```python
from build123d import *

# Parameters (mm, degrees)
ESQUISSE1_W              = 60
ESQUISSE1_H              = 89
BOSS_EXTRU_1_DEPTH       = 11.5
ESQUISSE2_W              = 15
ESQUISSE2_H              = 1.6
ENL_V_MAT_EXTRU_1_DEPTH  = 55.886246
ENL_V_MAT_EXTRU_2_REACH  = 94.584
ESQUISSE4_W              = 15
ESQUISSE4_H              = 9.9
ENL_V_MAT_EXTRU_3_REACH  = 75.647
ESQUISSE5_W              = 85.8
ESQUISSE5_H              = 9.9
ENL_V_MAT_EXTRU_4_REACH  = 75.647
ESQUISSE6_W              = 9.9
ESQUISSE6_H              = 85.8
ENL_V_MAT_EXTRU_5_REACH  = 76.922
ESQUISSE7_W              = 7
ESQUISSE7_H              = 10
ENL_V_MAT_EXTRU_6_REACH  = 76.922
ESQUISSE8_W              = 7
ESQUISSE8_H              = 18
ENL_V_MAT_EXTRU_7_REACH  = 96.096
ESQUISSE9_W              = 17.5
ESQUISSE9_H              = 7.5
ENL_V_MAT_EXTRU_8_REACH  = 96.096
ESQUISSE10_W             = 16
ESQUISSE10_H             = 7.5
ENL_V_MAT_EXTRU_9_REACH  = 96.096
ESQUISSE11_W             = 16
ESQUISSE11_H             = 7.5
ENL_V_MAT_EXTRU_10_REACH = 76.922
ESQUISSE12_W             = 7
ESQUISSE12_H             = 8.5
ESQUISSE23_W             = 2
ESQUISSE23_H             = 7.5
BOSS_EXTRU_5_DEPTH       = 7.5
ESQUISSE24_W             = 7.5
ESQUISSE24_H             = 2
BOSS_EXTRU_6_DEPTH       = 7.5
ESQUISSE25_W             = 2
ESQUISSE25_H             = 7.5
BOSS_EXTRU_7_DEPTH       = 8.1
ESQUISSE26_W             = 2
ESQUISSE26_H             = 7.5
BOSS_EXTRU_8_DEPTH       = 7.5
ESQUISSE28_W             = 1.25
ESQUISSE28_H             = 7
ESQUISSE29_W             = 1.25
ESQUISSE29_H             = 7
ESQUISSE30_W             = 1.25
ESQUISSE30_H             = 7
ESQUISSE31_W             = 1.25
ESQUISSE31_H             = 7
CONG_1_R                 = 2
CHANFREIN1_SIZE          = 0.3
CONG_2_R                 = 0.5
CONG_9_R                 = 2.5


with BuildPart() as part:
    # Esquisse1 → Boss.-Extru.1 (new body)
    with BuildSketch(Plane.XY.offset(5.75)):
        Rectangle(ESQUISSE1_W, ESQUISSE1_H)
    extrude(amount=-BOSS_EXTRU_1_DEPTH)

    # Esquisse2 → Enlèv. mat.-Extru.1 (cut, through all)
    with BuildSketch(Plane(origin=(0, 0, -5.75), x_dir=(-1, 0, 0), z_dir=(0, 0, -1))):
        with Locations((0, 43.7)):
            Rectangle(ESQUISSE2_W, ESQUISSE2_H)
    extrude(amount=-ENL_V_MAT_EXTRU_1_DEPTH, mode=Mode.SUBTRACT)

    # Esquisse4 → Enlèv. mat.-Extru.2 (cut, up to next)
    with BuildSketch(Plane.XZ.offset(42.9), mode=Mode.PRIVATE) as enl_v_mat_extru_2_sk1:
        with Locations((0, 0.8)):
            Rectangle(ESQUISSE4_W, ESQUISSE4_H)
    enl_v_mat_extru_2_tool1 = extrude(enl_v_mat_extru_2_sk1.sketch, amount=-ENL_V_MAT_EXTRU_2_REACH, mode=Mode.PRIVATE) & part.part
    add(enl_v_mat_extru_2_tool1.solids().sort_by_distance((0, -42.9, 0.8))[0], mode=Mode.SUBTRACT)

    # Esquisse5 → Enlèv. mat.-Extru.3 (cut, up to next)
    with BuildSketch(Plane(origin=(-28.4, 0, 0), x_dir=(0, -1, 0), z_dir=(-1, 0, 0)), mode=Mode.PRIVATE) as enl_v_mat_extru_3_sk1:
        with Locations((0, 0.8)):
            Rectangle(ESQUISSE5_W, ESQUISSE5_H)
    enl_v_mat_extru_3_tool1 = extrude(enl_v_mat_extru_3_sk1.sketch, amount=-ENL_V_MAT_EXTRU_3_REACH, mode=Mode.PRIVATE) & part.part
    add(enl_v_mat_extru_3_tool1.solids().sort_by_distance((-28.4, 0, 0.8))[0], mode=Mode.SUBTRACT)

    # Esquisse6 → Enlèv. mat.-Extru.4 (cut, up to next)
    with BuildSketch(Plane(origin=(28.4, 0, 0), x_dir=(0, 0, -1), z_dir=(1, 0, 0)), mode=Mode.PRIVATE) as enl_v_mat_extru_4_sk1:
        with Locations((-0.8, 0)):
            Rectangle(ESQUISSE6_W, ESQUISSE6_H)
    enl_v_mat_extru_4_tool1 = extrude(enl_v_mat_extru_4_sk1.sketch, amount=-ENL_V_MAT_EXTRU_4_REACH, mode=Mode.PRIVATE) & part.part
    add(enl_v_mat_extru_4_tool1.solids().sort_by_distance((28.4, 0, 0.8))[0], mode=Mode.SUBTRACT)

    # Esquisse7 → Enlèv. mat.-Extru.5 (cut, up to next)
    with BuildSketch(Plane.ZY.offset(30), mode=Mode.PRIVATE) as enl_v_mat_extru_5_sk1:
        with Locations((2.25, 32)):
            Rectangle(ESQUISSE7_W, ESQUISSE7_H)
    enl_v_mat_extru_5_tool1 = extrude(enl_v_mat_extru_5_sk1.sketch, amount=-ENL_V_MAT_EXTRU_5_REACH, mode=Mode.PRIVATE) & part.part
    add(enl_v_mat_extru_5_tool1.solids().sort_by_distance((-30, 32, 2.25))[0], mode=Mode.SUBTRACT)

    # Esquisse8 → Enlèv. mat.-Extru.6 (cut, up to next)
    with BuildSketch(Plane.ZY.offset(30), mode=Mode.PRIVATE) as enl_v_mat_extru_6_sk1:
        with Locations((2.25, 10.5)):
            Rectangle(ESQUISSE8_W, ESQUISSE8_H)
    enl_v_mat_extru_6_tool1 = extrude(enl_v_mat_extru_6_sk1.sketch, amount=-ENL_V_MAT_EXTRU_6_REACH, mode=Mode.PRIVATE) & part.part
    add(enl_v_mat_extru_6_tool1.solids().sort_by_distance((-30, 10.5, 2.25))[0], mode=Mode.SUBTRACT)

    # Esquisse9 → Enlèv. mat.-Extru.7 (cut, up to next)
    with BuildSketch(Plane.XZ.offset(44.5), mode=Mode.PRIVATE) as enl_v_mat_extru_7_sk1:
        with Locations((-17.75, 2)):
            Rectangle(ESQUISSE9_W, ESQUISSE9_H)
    enl_v_mat_extru_7_tool1 = extrude(enl_v_mat_extru_7_sk1.sketch, amount=-ENL_V_MAT_EXTRU_7_REACH, mode=Mode.PRIVATE) & part.part
    add(enl_v_mat_extru_7_tool1.solids().sort_by_distance((-17.75, -44.5, 2))[0], mode=Mode.SUBTRACT)

    # Esquisse10 → Enlèv. mat.-Extru.8 (cut, up to next)
    with BuildSketch(Plane.XZ.offset(44.5), mode=Mode.PRIVATE) as enl_v_mat_extru_8_sk1:
        with Locations((1, 2)):
            Rectangle(ESQUISSE10_W, ESQUISSE10_H)
    enl_v_mat_extru_8_tool1 = extrude(enl_v_mat_extru_8_sk1.sketch, amount=-ENL_V_MAT_EXTRU_8_REACH, mode=Mode.PRIVATE) & part.part
    add(enl_v_mat_extru_8_tool1.solids().sort_by_distance((1, -44.5, 2))[0], mode=Mode.SUBTRACT)

    # Esquisse11 → Enlèv. mat.-Extru.9 (cut, up to next)
    with BuildSketch(Plane.XZ.offset(44.5), mode=Mode.PRIVATE) as enl_v_mat_extru_9_sk1:
        with Locations((19, 2)):
            Rectangle(ESQUISSE11_W, ESQUISSE11_H)
    enl_v_mat_extru_9_tool1 = extrude(enl_v_mat_extru_9_sk1.sketch, amount=-ENL_V_MAT_EXTRU_9_REACH, mode=Mode.PRIVATE) & part.part
    add(enl_v_mat_extru_9_tool1.solids().sort_by_distance((19, -44.5, 2))[0], mode=Mode.SUBTRACT)

    # Esquisse12 → Enlèv. mat.-Extru.10 (cut, up to next)
    with BuildSketch(Plane.ZY.offset(30), mode=Mode.PRIVATE) as enl_v_mat_extru_10_sk1:
        with Locations((2.25, -11)):
            Rectangle(ESQUISSE12_W, ESQUISSE12_H)
    enl_v_mat_extru_10_tool1 = extrude(enl_v_mat_extru_10_sk1.sketch, amount=-ENL_V_MAT_EXTRU_10_REACH, mode=Mode.PRIVATE) & part.part
    add(enl_v_mat_extru_10_tool1.solids().sort_by_distance((-30, -11, 2.25))[0], mode=Mode.SUBTRACT)

    # Esquisse23 → Boss.-Extru.5 (add)
    with BuildSketch(Plane(origin=(-28.4, 0, 0), x_dir=(0, 0, -1), z_dir=(1, 0, 0))):
        with Locations((3.15, 39.15)):
            Rectangle(ESQUISSE23_W, ESQUISSE23_H)
    extrude(amount=BOSS_EXTRU_5_DEPTH)

    # Esquisse24 → Boss.-Extru.6 (add)
    with BuildSketch(Plane.XZ.offset(-42.9)):
        with Locations((24.65, -3.15)):
            Rectangle(ESQUISSE24_W, ESQUISSE24_H)
    extrude(amount=BOSS_EXTRU_6_DEPTH)

    # Esquisse25 → Boss.-Extru.7 (add)
    with BuildSketch(Plane.ZY.offset(-28.4)):
        with Locations((-3.15, -18.85)):
            Rectangle(ESQUISSE25_W, ESQUISSE25_H)
    extrude(amount=BOSS_EXTRU_7_DEPTH)

    # Esquisse26 → Boss.-Extru.8 (add)
    with BuildSketch(Plane(origin=(-28.4, 0, 0), x_dir=(0, 0, -1), z_dir=(1, 0, 0))):
        with Locations((3.15, -18.85)):
            Rectangle(ESQUISSE26_W, ESQUISSE26_H)
    extrude(amount=BOSS_EXTRU_8_DEPTH)

    # Esquisse28 → Révolution1 (revolve)
    with BuildSketch(Plane(origin=(0, -18.85, 0), x_dir=(1, 0, 0), z_dir=(0, 1, 0))):
        with Locations((24.975, -1.35)):
            Rectangle(ESQUISSE28_W, ESQUISSE28_H)
    revolve(axis=Axis((24.35, -18.85, -2.15), (0, 0, 1)))

    # Esquisse29 → Révolution2 (revolve)
    with BuildSketch(Plane(origin=(0, 39.15, 0), x_dir=(1, 0, 0), z_dir=(0, 1, 0))):
        with Locations((24.975, -1.35)):
            Rectangle(ESQUISSE29_W, ESQUISSE29_H)
    revolve(axis=Axis((24.35, 39.15, -2.15), (0, 0, 1)))

    # Esquisse30 → Révolution3 (revolve)
    with BuildSketch(Plane(origin=(0, 39.15, 0), x_dir=(1, 0, 0), z_dir=(0, 1, 0))):
        with Locations((-24.025, -1.35)):
            Rectangle(ESQUISSE30_W, ESQUISSE30_H)
    revolve(axis=Axis((-24.65, 39.15, -2.15), (0, 0, 1)))

    # Esquisse31 → Révolution4 (revolve)
    with BuildSketch(Plane(origin=(0, -18.85, 0), x_dir=(1, 0, 0), z_dir=(0, 1, 0))):
        with Locations((-24.025, -1.35)):
            Rectangle(ESQUISSE31_W, ESQUISSE31_H)
    revolve(axis=Axis((-24.65, -18.85, -2.15), (0, 0, 1)))

    # Congé1
    cong_1_edges = [part.edges().sort_by_distance(p)[0] for p in [
        (30, -44.5, 0),
        (-30, -44.5, 0),
        (-30, 44.5, 0),
        (30, 44.5, 0),
    ]]
    fillet(cong_1_edges, radius=CONG_1_R)

    # Chanfrein1
    chanfrein1_edges = [part.edges().sort_by_distance(p)[0] for p in [
        (23.1, -18.85, 4.85),
        (23.1, 39.15, 4.85),
        (-25.9, 39.15, 4.85),
        (-25.9, -18.85, 4.85),
    ]]
    chamfer(chanfrein1_edges, length=CHANFREIN1_SIZE)

    # Congé2
    cong_2_edges = [part.edges().sort_by_distance(p)[0] for p in [
        (-17.75, 44.5, -5.75),
        (30, 0, -5.75),
        (17.75, 44.5, -5.75),
        (0, -44.5, -5.75),
        (-30, 0, -5.75),
        (-29.414213562, -43.914213562, -5.75),
        (29.414213562, -43.914213562, -5.75),
        (-29.414213562, 43.914213562, -5.75),
        (29.414213562, 43.914213562, -5.75),
    ]]
    fillet(cong_2_edges, radius=CONG_2_R)

    # Congé9
    cong_9_edges = [part.edges().sort_by_distance(p)[0] for p in [
        (-28.4, 35.4, -3.15),
        (-20.9, 35.4, -3.15),
        (-20.9, 42.9, -3.15),
        (20.9, 42.9, -3.15),
        (20.9, 35.4, -3.15),
        (28.4, 35.4, -3.15),
        (28.4, -22.6, -3.15),
        (28.4, -15.1, -3.15),
        (20.3, -22.6, -3.15),
        (20.3, -15.1, -3.15),
        (-28.4, -22.6, -3.15),
        (-28.4, -15.1, -3.15),
        (-20.9, -22.6, -3.15),
        (-20.9, -15.1, -3.15),
    ]]
    fillet(cong_9_edges, radius=CONG_9_R)


solid = part.part
```
For this review, take the finished solid that the model builds, in its own axes (mm). A direction names the side the tool comes from. Coordinates: 2 decimals unless noted, no trailing zeros. Write each loop counter-clockwise with the first axis right and the second up, starting at its lowest first coordinate (ties: lowest second). Pieces come first, ordered by that corner, then holes. Notation, with made-up numbers: (-32, 28.25) - (-11, 28.25) arc R17 ccw to (-11, 46.25) - close; hole circle Ø4 at (71.5, 20.25). An arc over 180 degrees is marked (long way). Answer in a Markdown table with one row per item. Add a question column.
Q1. We need section C-C, the plane z = 1.75. Count the separate pieces of the cut face and the enclosed holes in it, and give its area (3 significant figures).
Q2. We need section B-B, the plane x = 13.5. State the section outline as (y, z) points, and give its area (3 significant figures).
Q3. Draft analysis for pull direction X (two halves, no side actions). For faces 3 (the flat face through (30, -1, 0)), 4 (the flat face through (-25, 39, 4.85)), 5 (the flat face through (18, 44.5, 0)), state which applies: +X half, -X half, draft (parallel to the pull), parting line (faces both ways), or undercut.
Q4. We need section D-D, the plane x = 24.35. State the section outline as (y, z) points, and give its area (3 significant figures).
Q5. For probe 1 along X at (y, z) = (16, -2.5); probe 2 along Y at (x, z) = (17, -4); probe 3 along Y at (x, z) = (-2.5, -4), list the stretches that pass through material, from the lowest coordinate up.
Q6. Tool access review of faces 1 (the cylindrical face through (-29.43, 43.9, 0.17)), 2 (the flat face through (20.9, 39, -3)): name each direction out of +Z, -Z, +X, -X, +Y, -Y from which nothing blocks a thin tool from reaching the whole face with its end or side.
Q7. For P1, Ø1.5, axis at x = -24, y = 39.5, coming from the +Z side; P2, Ø0.5, axis at x = -29.5, z = 2.5, coming from the +Y side; P3, Ø0.8, axis at x = -29.5, z = 0.5, coming from the -Y side, all flat-tipped, find the tip position at first contact; note any pin that passes through.
Q8. We need section A-A, the plane y = -27.5. State the section outline as (x, z) points, and give its area (3 significant figures).
Answer list:
| question | item | result |
|---|---|---|
| 1 | separate pieces | 11 |
| 1 | enclosed holes | 0 |
| 1 | area | 321 mm2 |
| 2 | outline | (-44.5, -5.25) arc R0.5 ccw to (-44, -5.75) - (44, -5.75) arc R0.5 ccw to (44.5, -5.25) - (44.5, 5.75) - (42.9, 5.75) - (42.9, -4.15) - (-42.9, -4.15) - (-42.9, -1.75) - (-44.5, -1.75) - close |
| 2 | area | 162 mm2 |
| 3 | face 3 | +X half |
| 3 | face 4 | undercut |
| 3 | face 5 | draft |
| 4 | outline | (-44.5, -5.25) arc R0.5 ccw to (-44, -5.75) - (44, -5.75) arc R0.5 ccw to (44.5, -5.25) - (44.5, 5.75) - (42.9, 5.75) - (42.9, -2.15) - (40.4, -2.15) - (40.4, 4.55) - (40.1, 4.85) - (38.2, 4.85) - (37.9, 4.55) - (37.9, -2.15) - (35.4, -2.15) - (35.4, -4.15) - (-15.1, -4.15) - (-15.1, -2.15) - (-17.6, -2.15) - (-17.6, 4.55) - (-17.9, 4.85) - (-19.8, 4.85) - (-20.1, 4.55) - (-20.1, -2.15) - (-22.6, -2.15) - (-22.6, -4.15) - (-42.9, -4.15) - (-42.9, -1.75) - (-44.5, -1.75) - close |
| 4 | area | 227 mm2 |
| 5 | probe 1 | x = -30 to -28.4, 28.4 to 30 |
| 5 | probe 2 | y = -44.5 to -42.9, 42.9 to 44.5 |
| 5 | probe 3 | y = -44.5 to -42.9 |
| 6 | face 1 | +Z, -Z, -X, +Y |
| 6 | face 2 | +Z |
| 7 | P1 | stops at z = 4.85 |
| 7 | P2 | stops at y = 44.06 |
| 7 | P3 | stops at y = -44.17 |
| 8 | outline | (-30, -5.25) arc R0.5 ccw to (-29.5, -5.75) - (29.5, -5.75) arc R0.5 ccw to (30, -5.25) - (30, 5.75) - (28.4, 5.75) - (28.4, -4.15) - (-28.4, -4.15) - (-28.4, 5.75) - (-30, 5.75) - close |
| 8 | area | 128 mm2 |
